Part model, mm, in its own coordinate system. Round coordinates to 2 decimals unless told otherwise and drop trailing zeros. Order: outer loops, then holes, each group sorted by start corner. A loop starts at its lowest first (then second) coordinate and runs counter-clockwise, first axis right, second up. Notation, with made-up numbers: (22, 69) - (46, 69) arc R24 cw to (46, 84) - close; hole circle Ø3 at (52.5, 69.5). An arc over 180 degrees is marked (long way). Return JSON: item names as keys, results as strings. Group by question number.
Item 1: Saw through at C-C on x = -0.45. List the corners of the cut face in (y, z) (3 decimals).
Item 2: Probe probe 1 along Y at (x, z) = (-0.55, 0) (3 decimals); probe 2 along Y at (x, z) = (-0.4, -1.25). List the from-to ranges inside material, lowest first.
Item 3: Saw through at A-A on z = 0. List the corners of the cut face in (x, y) (3 decimals).
Item 4: Two-plate mould, pull along Y, no slides. Class faces 1 (the face through (0, 3, -3)), 2 (the face through (-0.494, -1.032, 3.276)), 3 (the face through (-0.49, -1.95, 6.2)): released by +Y, released by -Y, zero draft, split by the parting line, or undercut.
```python
from build123d import *

# Parameters (mm, degrees)
SKETCH1_W     = 1.75
SKETCH1_H     = 3.065
CHAMFER1_SIZE = 0.1


# Read off the part's stored shape, not the designer's step: Move Face1
with BuildPart() as part:
    # Sketch1 → Base-Revolve (revolve)
    with BuildSketch(Plane.XY, mode=Mode.PRIVATE) as base_revolve_sk:
        with Locations((-0.875, 4.9675)):
            Rectangle(SKETCH1_W, SKETCH1_H)
    revolve(base_revolve_sk.sketch.rotate(Axis((-34.925, 0, 0), (1, 0, 0)), 90), axis=Axis((-34.925, 0, 0), (1, 0, 0)))

    # Chamfer1
    chamfer1_edges = [part.edges().sort_by_distance(p)[0] for p in [
        (-1.75, 0, -3.435),
        (-1.75, 0, -6.5),
        (0, 0, -6.5),
        (0, 0, -3.435),
    ]]
    chamfer(chamfer1_edges, length=CHAMFER1_SIZE)

    # Move Face1 outline → Move Face1 (revolve, cut)
    with BuildSketch(Plane.YX):
        Polygon((6.4, -1), (3.535, -1), (3.435, -0.9), (3.435, -1.65), (3.535, -1.75), (6.4, -1.75), (6.5, -1.65), (6.5, -0.9), align=None)
    revolve(axis=Axis((0, 0, 0), (1, 0, 0)), mode=Mode.SUBTRACT)


solid = part.part
```
Filled in:
{
 "1": {"outline": "circle Ø13 at (0, 0); hole circle Ø6.87 at (0, 0)"},
 "2": {"probe 1": "y = -6.5 to -3.435, 3.435 to 6.5", "probe 2": "y = -6.38 to -3.2, 3.2 to 6.38"},
 "3": {"outline": "(-1, -6.4) - (-0.9, -6.5) - (-0.1, -6.5) - (0, -6.4) - (0, -3.535) - (-0.1, -3.435) - (-0.9, -3.435) - (-1, -3.535) - close; (-1, 3.535) - (-0.9, 3.435) - (-0.1, 3.435) - (0, 3.535) - (0, 6.4) - (-0.1, 6.5) - (-0.9, 6.5) - (-1, 6.4) - close"},
 "4": {"face 1": "zero draft", "face 2": "undercut", "face 3": "split by the parting line"}
}
